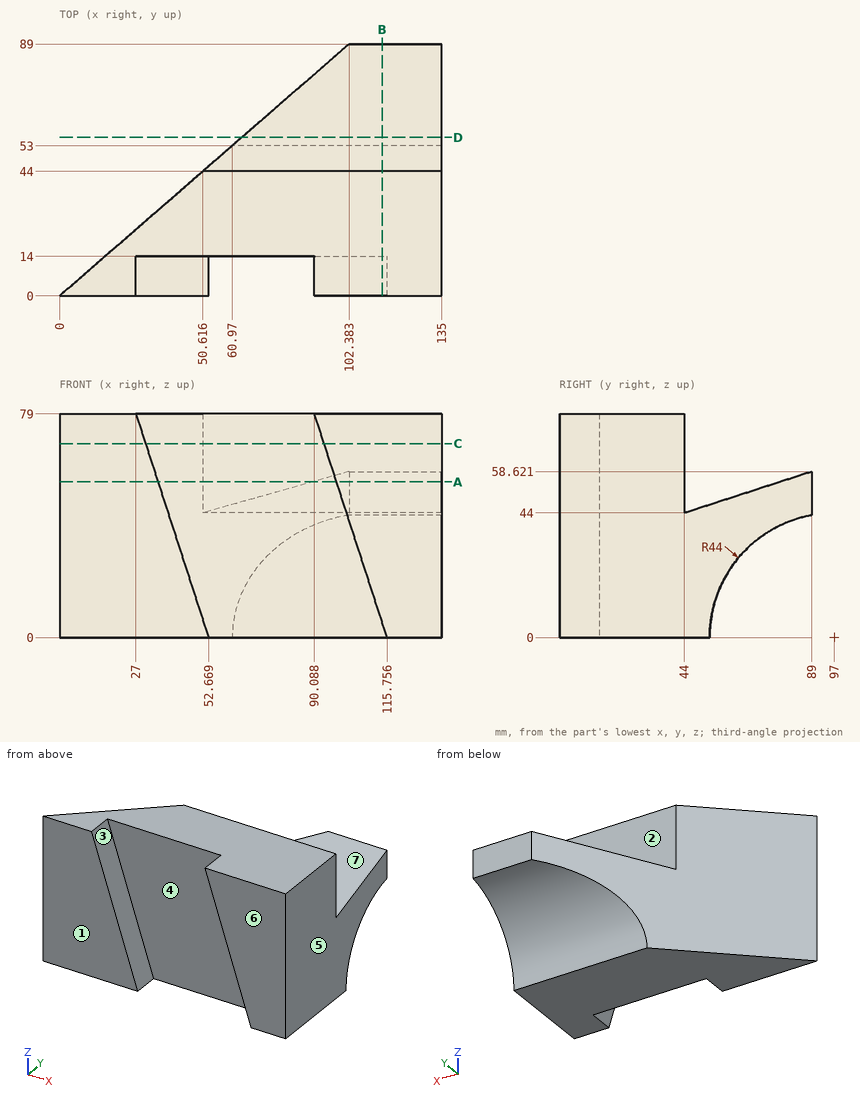
Drawing for the job (mm, zero at the part's lowest x, y, z). A direction names the side the tool comes from. Round coordinates to 2 decimals unless told otherwise and drop trailing zeros. Order: outer loops, then holes, each group sorted by start corner. A loop starts at its lowest first (then second) coordinate and runs counter-clockwise, first axis right, second up. Notation, with made-up numbers: (-12.75, 81) -> (1.25, 81) arc R30 cw to (1.25, 111) -> close; hole circle Ø8 at (11.25, -21.5). An arc over 180 degrees is marked (long way). Write item = value, one per line. Start each with the question number.
(1) Which spindle directions (+Z, -Z, +X, -X, +Y, -Y) get a long thin tool onto all of the face, cutting with end or side? Do the marked faces 1, 2, 3 and 4. Say none if no direction does.
(2) Pull direction Y, two halves, no side cores. Call the marked faces 5, 6 and 7: released by +Y, released by -Y, zero draft, split by the parting line, or undercut.
(3) Probe line 1 (X direction, y = 4.5, z = 52.5) (1 decimal); line 2 (Y direction, x = 91, z = 21.5); line 3 (X direction, y = 33.5, z = 24.5) (1 decimal). List the from-to ranges inside material, lowest first. Write a range as [from, to].
(4) Pin check, flat tips, straight feed: P1, Ø8, axis at x = 95.5, z = 10.5, coming from the -Y side; P2, Ø12, axis at y = 18.5, z = 36, coming from the -X side; P3, Ø6, axis at x = 37.5, z = 49.5, coming from the +Y side (1 decimal). Stop position of each tip, or through.
(5) Cut at B-B, the plane x = 114. List the corners of the cut face in (y, z) (1 decimal), then the cut area to 3 significant figures.
(6) Cut at C-C, the plane z = 68.5. List the corners of the cut face in (x, y).
(7) Cut at D-D, the plane y = 56. List the corners of the cut face in (x, z), then the cut area to 3 significant figures.
(8) Cut at A-A, the plane z = 55. List the corners of the cut face in (x, y) (1 decimal), then the cut area to 3 significant figures.
Model answer:
q1.face_1 = +Z, -Z, +X, -X, -Y
q1.face_2 = +Z, +X, -X
q1.face_3 = +Z, -Y
q1.face_4 = -Y
q2.face_5 = zero draft
q2.face_6 = released by -Y
q2.face_7 = undercut
q3.line_1 = [5.2, 35.6], [98.7, 135]
q3.line_2 = [14, 58.61]
q3.line_3 = [38.5, 135]
q4.P1 = 14
q4.P2 = 14.38
q4.P3 = 35.2
q5.outline = (0, 5.4) -> (14, 5.4) -> (14, 0) -> (53, 0) arc R44 cw to (89, 43.3) -> (89, 58.6) -> (44, 44) -> (44, 79) -> (0, 79) -> close
q5.area = 4,540 mm2
q6.outline = (0, 0) -> (30.41, 0) -> (30.41, 14) -> (93.5, 14) -> (93.5, 0) -> (135, 0) -> (135, 44) -> (50.62, 44) -> close
q7.outline = (64.42, 15.97) -> (135, 15.97) -> (135, 47.9) -> (64.42, 47.9) -> close
q7.area = 2,250 mm2
q8.outline = (0, 0) -> (34.8, 0) -> (34.8, 14) -> (97.9, 14) -> (97.9, 0) -> (135, 0) -> (135, 44) -> (50.6, 44) -> close; (89.6, 77.9) -> (135, 77.9) -> (135, 89) -> (102.4, 89) -> close
q8.area = 4,380 mm2
